```python
from build123d import *

# Parameters (mm, degrees)
SKETCH1_R           = 22.5
SKETCH1_W           = 10
SKETCH1_H           = 15
SKETCH1_W_2         = 45
SKETCH1_H_2         = 22.5
BOSS_EXTRUDE2_DEPTH = 25
SKETCH3_R           = 17.5
SKETCH3_W           = 4
SKETCH3_H           = 35
CUT_EXTRUDE2_DEPTH  = 25
SKETCH5_R           = 2.513863355
CUT_EXTRUDE3_DEPTH  = 60.581876439
SKETCH7_R           = 1.75
CUT_EXTRUDE4_DEPTH  = 48.762433046


with BuildPart() as part:
    # Sketch1 → Boss-Extrude2 (new body)
    with BuildSketch(Plane.XY):
        Circle(SKETCH1_R)
        with Locations((0, 22.5)):
            Rectangle(SKETCH1_W, SKETCH1_H)
        with Locations((0, -11.25)):
            Rectangle(SKETCH1_W_2, SKETCH1_H_2)
    extrude(amount=BOSS_EXTRUDE2_DEPTH)

    # Sketch3 → Cut-Extrude2 (cut)
    with BuildSketch(Plane.XY.offset(25)):
        Circle(SKETCH3_R)
        with Locations((0, 17.5)):
            Rectangle(SKETCH3_W, SKETCH3_H)
    extrude(amount=-CUT_EXTRUDE2_DEPTH, mode=Mode.SUBTRACT)

    # Sketch5 → Cut-Extrude3 (cut, through all)
    with BuildSketch(Plane.ZY.offset(22.5)):
        with Locations((19, -16.5)):
            Circle(SKETCH5_R)
    extrude(amount=-CUT_EXTRUDE3_DEPTH, mode=Mode.SUBTRACT)

    # Sketch7 → Cut-Extrude4 (cut, through all)
    with BuildSketch(Plane.ZY.offset(5)):
        with Locations(Location((3.5, 25.968705484, 0), (0, 0, 270))):
            Circle(SKETCH7_R)
        with Locations(Location((21.5, 25.968705484, 0), (0, 0, 270))):
            Circle(SKETCH7_R)
    extrude(amount=-CUT_EXTRUDE4_DEPTH, mode=Mode.SUBTRACT)


solid = part.part
```
Source: CAD feature listing. Evaluate the final solid. Frame: model axes, mm. A direction names the side the tool comes from. Round coordinates to 2 decimals unless told otherwise and drop trailing zeros. Loops run counter-clockwise (first coordinate to the right, second up) from the corner with the lowest first, then second, coordinate; pieces in that order, holes last.
(1) Section query C-C (z = 3.5). Output: boundary loops of the cut face in (x, y), and give its area (3 significant figures).
From the geometry:
outline: (-22.5, -22.5) - (22.5, -22.5) - (22.5, 0) arc R22.5 ccw to (5, 21.94) - (5, 24.22) - (2, 24.22) - (2, 17.39) arc R17.5 cw (long way) to (-2, 17.39) - (-2, 24.22) - (-5, 24.22) - (-5, 21.94) arc R22.5 ccw to (-22.5, 0) - close; (-5, 27.72) - (-2, 27.72) - (-2, 30) - (-5, 30) - close; (2, 27.72) - (5, 27.72) - (5, 30) - (2, 30) - close
area: 851 mm2
(2) Section query B-B (y = -16.5). Output: boundary loops of the cut face in (x, z), and give its area (3 significant figures).
From the geometry:
outline: (-22.5, 0) - (-5.83, 0) - (-5.83, 16.49) - (-22.5, 16.49) - close; (-22.5, 21.51) - (-5.83, 21.51) - (-5.83, 25) - (-22.5, 25) - close; (5.83, 0) - (22.5, 0) - (22.5, 16.49) - (5.83, 16.49) - close; (5.83, 21.51) - (22.5, 21.51) - (22.5, 25) - (5.83, 25) - close
area: 666 mm2
(3) Access query for faces 4 (the flat face through (-5, 26, 12)), 5 (the flat face through (2, -18, 25)). Directions: +Z, -Z, +X, -X, +Y, -Y. A direction counts if a zero-diameter tool reaches every point of the face in a straight line with its end or side. Return the directions, or none.
From the geometry:
face 4: +Z, -Z, -X, +Y
face 5: +Z, +X, -X, +Y, -Y
(4) Material intervals for probe 1 along X at (y, z) = (0.5, 23.25); probe 2 along X at (y, z) = (22.5, 9.25); probe 3 along Z at (x, y) = (18.5, -16.5), sorted ascending.
From the geometry:
probe 1: x = -22.49 to -17.49, 17.49 to 22.49
probe 2: x = -5 to -2, 2 to 5
probe 3: z = 0 to 16.49, 21.51 to 25
(5) Section query A-A (x = -15.5). Output: boundary loops of the cut face in (y, z), and give its area (3 significant figures).
From the geometry:
outline: (-22.5, 0) - (-8.12, 0) - (-8.12, 25) - (-22.5, 25) - close; (8.12, 0) - (16.31, 0) - (16.31, 25) - (8.12, 25) - close; hole circle Ø5.03 at (-16.5, 19)
area: 544 mm2
(6) Section query D-D (y = 6). Output: boundary loops of the cut face in (x, z), and give its area (3 significant figures).
From the geometry:
outline: (-21.69, 0) - (-16.44, 0) - (-16.44, 25) - (-21.69, 25) - close; (16.44, 0) - (21.69, 0) - (21.69, 25) - (16.44, 25) - close
area: 262 mm2
(7) Pull-direction query (X, two-part tool) for faces 1 (the flat face through (2, 24, 13)), 2 (the flat face through (5, 26, 12)), 3 (the cylindrical face through (3.479, 25.028, 22.976)); classes: +X half, -X half, draft (parallel to the pull), parting line (faces both ways), or undercut.
From the geometry:
face 1: undercut
face 2: +X half
face 3: draft
(8) Contact query for flat-ended pins moving along their axis: pin 1 Ø4 at (y, z) = (25.97, 3.5) entering from +X; pin 2 Ø10 at (y, z) = (21.5, 15.5) entering from +X; pin 3 Ø10 at (y, z) = (7, 9) entering from -X. Output: stop coordinate, or through.
From the geometry:
pin 1: stops at x = 5
pin 2: stops at x = 15.3
pin 3: stops at x = -22.41
